```python
from build123d import *

# Parameters (mm, degrees)
BOSS_EXTRUDE1_DEPTH = 3
BOSS_EXTRUDE4_DEPTH = 10
BOSS_EXTRUDE5_DEPTH = 2


with BuildPart() as part:
    # Sketch2 → Boss-Extrude1 (new body)
    with BuildSketch(Plane(origin=(0, 3, 0), x_dir=(1, 0, 0), z_dir=(0, 0, 1))):
        with BuildLine():
            Line((-56.625, -30), (56.625, -30))
            Line((56.625, -30), (56.625, -15.644630074))
            ThreePointArc((56.625, -15.644630074), (56.398076263, -14.603897494), (55.758500558, -13.752098455))
            Line((55.758500558, -13.752098455), (44.005193779, -3.607468381))
            ThreePointArc((44.005193779, -3.607468381), (43.243091796, -3.156783296), (42.371693222, -3))
            Line((42.371693222, -3), (-42.371693222, -3))
            ThreePointArc((-42.371693222, -3), (-43.243091796, -3.156783296), (-44.005193779, -3.607468381))
            Line((-44.005193779, -3.607468381), (-55.758500558, -13.752098455))
            ThreePointArc((-55.758500558, -13.752098455), (-56.398076263, -14.603897494), (-56.625, -15.644630074))
            Line((-56.625, -15.644630074), (-56.625, -30))
        make_face()
    extrude(amount=BOSS_EXTRUDE1_DEPTH)

    # Sketch5 → Boss-Extrude4 (add)
    with BuildSketch(Plane.XY.offset(3)):
        with BuildLine():
            Line((55.625, -26), (55.625, -12.644630074))
            ThreePointArc((55.625, -12.644630074), (55.488845758, -12.020190526), (55.105100335, -11.509111102))
            Line((55.105100335, -11.509111102), (43.351793556, -1.364481029))
            ThreePointArc((43.351793556, -1.364481029), (42.894532367, -1.094069977), (42.371693222, -1))
            Line((42.371693222, -1), (-42.371693222, -1))
            ThreePointArc((-42.371693222, -1), (-42.894532367, -1.094069977), (-43.351793556, -1.364481029))
            Line((-43.351793556, -1.364481029), (-55.105100335, -11.509111102))
            ThreePointArc((-55.105100335, -11.509111102), (-55.488845758, -12.020190526), (-55.625, -12.644630074))
            Line((-55.625, -12.644630074), (-55.625, -26))
            Line((-55.625, -26), (55.625, -26))
        make_face()
    extrude(amount=BOSS_EXTRUDE4_DEPTH)

    # Sketch6 → Boss-Extrude5 (add)
    with BuildSketch(Plane(origin=(0, 0, 0), x_dir=(-1, 0, 0), z_dir=(0, 0, -1))):
        with BuildLine():
            Line((-62.2875, -12.644630074), (-62.2875, -28.435536993))
            Line((-62.2875, -28.435536993), (62.2875, -28.435536993))
            Line((62.2875, -28.435536993), (62.2875, -12.644630074))
            ThreePointArc((62.2875, -12.644630074), (62.037883889, -11.499824236), (61.334350613, -10.562845293))
            Line((61.334350613, -10.562845293), (48.405713157, 0.596247788))
            ThreePointArc((48.405713157, 0.596247788), (47.567400976, 1.092001382), (46.608862544, 1.264463007))
            Line((46.608862544, 1.264463007), (-46.608862544, 1.264463007))
            ThreePointArc((-46.608862544, 1.264463007), (-47.567400976, 1.092001382), (-48.405713157, 0.596247788))
            Line((-48.405713157, 0.596247788), (-61.334350613, -10.562845293))
            ThreePointArc((-61.334350613, -10.562845293), (-62.037883889, -11.499824236), (-62.2875, -12.644630074))
        make_face()
    extrude(amount=BOSS_EXTRUDE5_DEPTH)


solid = part.part
```
Input: part model. Units: mm. Frame: model coordinates. A direction names the side the tool comes from. Round coordinates to 2 decimals unless told otherwise and drop trailing zeros. Order: outer loops, then holes, each group sorted by start corner. A loop starts at its lowest first (then second) coordinate and runs counter-clockwise, first axis right, second up. Notation, with made-up numbers: (-24.75, 57.5) - (32.25, 57.5) arc R16 ccw to (32.25, 79.5) - close; hole circle Ø4 at (72, 50). An arc over 180 degrees is marked (long way). Answer in a Markdown table with one row per item.
Item 1: Section query A-A (z = 7.5). Return the cut outline in (x, y) (3 decimals).
Model answer:
| item | result |
|---|---|
| outline | (-55.625, -26) - (55.625, -26) - (55.625, -12.645) arc R1.5 ccw to (55.105, -11.509) - (43.352, -1.364) arc R1.5 ccw to (42.372, -1) - (-42.372, -1) arc R1.5 ccw to (-43.352, -1.364) - (-55.105, -11.509) arc R1.5 ccw to (-55.625, -12.645) - close |
Item 2: Section query C-C (y = -14.5). Return the cut outline in (x, z) (1 decimal).
Model answer:
| item | result |
|---|---|
| outline | (-62.3, -2) - (62.3, -2) - (62.3, 0) - (56.6, 0) - (56.6, 3) - (55.6, 3) - (55.6, 13) - (-55.6, 13) - (-55.6, 3) - (-56.6, 3) - (-56.6, 0) - (-62.3, 0) - close |
Item 3: Line query: line 1 (X direction, y = -25.75, z = 10.25) (3 decimals); line 2 (Z direction, x = -57, y = -16.75); line 3 (Y direction, x = 14.5, z = 10). Output: solid intervals per line, ascending.
Model answer:
| item | result |
|---|---|
| line 1 | x = -55.625 to 55.625 |
| line 2 | z = -2 to 0 |
| line 3 | y = -26 to -1 |
Item 4: Pin query (flat end, axial travel): pin 1 (6 mm diameter, centred on y = -25, z = 10.5, fed in from +X) (3 decimals); pin 2 (3 mm diameter, centred on y = -19.5, z = 8.5, fed in from -X) (3 decimals); pin 3 (1.5 mm diameter, centred on y = -20.5, z = 2, fed in from -X) (3 decimals). Return the tip coordinate at first contact, or that it passes through.
Model answer:
| item | result |
|---|---|
| pin 1 | stops at x = 55.625 |
| pin 2 | stops at x = -55.625 |
| pin 3 | stops at x = -56.625 |
Item 5: Section query B-B (x = -29.5). Return the cut outline in (y, z).
Model answer:
| item | result |
|---|---|
| outline | (-28.44, -2) - (1.26, -2) - (1.26, 0) - (0, 0) - (0, 3) - (-1, 3) - (-1, 13) - (-26, 13) - (-26, 3) - (-27, 3) - (-27, 0) - (-28.44, 0) - close |
Item 6: Reachability of faces 1 (the flat face through (55.625, -19, 8)), 2 (the flat face through (-1, -27, 1)), 3 (the flat face through (1, 0, 1)), 4 (the flat face through (-56.625, -20, 1)) from +Z, -Z, +X, -X, +Y, -Y: full face, straight path, thin tool, end or side. Return the list, or none.
Model answer:
| item | result |
|---|---|
| face 1 | +Z, +X, +Y, -Y |
| face 2 | +Z, +X, -X, -Y |
| face 3 | +Z, +X, -X, +Y |
| face 4 | +Z, -X, +Y, -Y |
